from build123d import *

# Parameters (mm, degrees)
SKETCH2_R            = 39.5
BOSS_EXTRUDE1_DEPTH  = 1
SKETCH4_R            = 41.25
BOSS_EXTRUDE2_DEPTH  = 1
SKETCH5_R            = 42
BOSS_EXTRUDE3_DEPTH  = 7
SKETCH6_R            = 35
BOSS_EXTRUDE4_DEPTH  = 7
BOSS_EXTRUDE5_DEPTH  = 3
CIRPATTERN1_COUNT    = 12
SKETCH8_R            = 15
BOSS_EXTRUDE6_DEPTH  = 10
SKETCH9_W            = 24
SKETCH9_H            = 40
BOSS_EXTRUDE7_DEPTH  = 42
BOSS_EXTRUDE8_START  = -24
BOSS_EXTRUDE8_DEPTH  = 24
SKETCH11_R           = 15
BOSS_EXTRUDE9_DEPTH  = 10
BOSS_EXTRUDE10_START = 10
SKETCH12_R           = 15
BOSS_EXTRUDE10_DEPTH = 10


with BuildPart() as part:
    # Sketch1 → Revolve1 (revolve)
    with BuildSketch(Plane.XY):
        with BuildLine():
            Line((0, 0), (-35, 0))
            ThreePointArc((-35, 0), (-39.657515479, -9.46062113), (-40, -20))
            Line((-40, -20), (0, -20))
            Line((0, -20), (0, 0))
        make_face()
    revolve(axis=Axis((0, 0, 0), (0, -1, 0)))

    # Sketch2 → Boss-Extrude1 (add)
    with BuildSketch(Plane.XZ.offset(20)):
        Circle(SKETCH2_R)
    extrude(amount=BOSS_EXTRUDE1_DEPTH)

    # Sketch3 → Revolve3 (revolve)
    with BuildSketch(Plane(origin=(0, 0, 0), x_dir=(0, 0, -1), z_dir=(1, 0, 0)), mode=Mode.PRIVATE) as revolve3_sk:
        with BuildLine():
            Line((0, -21), (-40, -21))
            ThreePointArc((-40, -21), (-42.384109041, -30.861589096), (-42, -41))
            Line((-42, -41), (0, -41))
            Line((0, -41), (0, -21))
        make_face()
    revolve(revolve3_sk.sketch.rotate(Axis((0, -21, 0), (0, -1, 0)), 90), axis=Axis((0, -21, 0), (0, -1, 0)))

    # Sketch4 → Boss-Extrude2 (add)
    with BuildSketch(Plane.XZ.offset(41)):
        with Locations(Location((0, 0, 0), (0, 0, 270))):
            Circle(SKETCH4_R)
    extrude(amount=BOSS_EXTRUDE2_DEPTH)

    # Sketch5 → Boss-Extrude3 (add)
    with BuildSketch(Plane.XZ.offset(42)):
        with Locations(Location((0, 0, 0), (0, 0, 270))):
            Circle(SKETCH5_R)
    extrude(amount=BOSS_EXTRUDE3_DEPTH)

    # Sketch6 → Boss-Extrude4 (add)
    with BuildSketch(Plane.XZ.offset(49)):
        with Locations(Location((0, 0, 0), (0, 0, 270))):
            Circle(SKETCH6_R)
    extrude(amount=BOSS_EXTRUDE4_DEPTH)

    # Sketch7 → Boss-Extrude5 (add)
    with BuildSketch(Plane.XZ.offset(49)):
        Polygon((36.25, 0), (37.375, -1.948557159), (39.625, -1.948557159), (40.75, 0), (39.625, 1.948557159), (37.375, 1.948557159), align=None)
        Polygon((37.952350269, 0.948557159), (37.404700538, 0), (37.952350269, -0.948557159), (39.047649731, -0.948557159), (39.595299462, 0), (39.047649731, 0.948557159), align=None, mode=Mode.SUBTRACT)
    boss_extrude5 = extrude(amount=BOSS_EXTRUDE5_DEPTH)

    # CirPattern1: Boss-Extrude5 ×12 about axis
    cirpattern1_axis = Axis((0, 0, 0), (0, 1, 0))
    for i in range(1, CIRPATTERN1_COUNT):
        add(boss_extrude5.rotate(cirpattern1_axis, i * 360 / CIRPATTERN1_COUNT))

    # Sketch8 → Boss-Extrude6 (add)
    with BuildSketch(Plane.XZ.offset(56)):
        with Locations(Location((0, 0, 0), (0, 0, 270))):
            Circle(SKETCH8_R)
    extrude(amount=BOSS_EXTRUDE6_DEPTH)

    # Sketch9 → Boss-Extrude7 (add)
    with BuildSketch(Plane(origin=(0, 0, 0), x_dir=(1, 0, 0), z_dir=(0, 1, 0))):
        Rectangle(SKETCH9_W, SKETCH9_H)
    extrude(amount=BOSS_EXTRUDE7_DEPTH)

    # Sketch10 → Boss-Extrude8 (add)
    with BuildSketch(Plane(origin=(12, 0, 0), x_dir=(0, 0, -1), z_dir=(1, 0, 0)).offset(BOSS_EXTRUDE8_START)):
        with BuildLine():
            Line((-20, 42), (20, 42))
            ThreePointArc((20, 42), (0, 62), (-20, 42))
        make_face()
    extrude(amount=BOSS_EXTRUDE8_DEPTH)

    # Sketch11 → Boss-Extrude9 (add)
    with BuildSketch(Plane(origin=(12, 0, 0), x_dir=(0, 0, -1), z_dir=(1, 0, 0))):
        with Locations(Location((0, 42, 0), (0, 0, 180))):
            Circle(SKETCH11_R)
    extrude(amount=BOSS_EXTRUDE9_DEPTH)

    # Sketch12 → Boss-Extrude10 (add)
    with BuildSketch(Plane.ZY.offset(12).offset(BOSS_EXTRUDE10_START)):
        with Locations((0, 42)):
            Circle(SKETCH12_R)
    extrude(amount=-BOSS_EXTRUDE10_DEPTH)


solid = part.part
The model under review builds one solid part; all positions refer to its coordinate system, in mm. A direction names the side the tool comes from. Coordinates: 2 decimals unless noted, no trailing zeros. Answer as a JSON object with one key per item and string values. Group by question number.
1. To check wall thickness, follow probe 1 along Y at (x, z) = (-9, 0); probe 2 along Y at (x, z) = (32.5, -12); probe 3 along X at (y, z) = (8, -1.5). State the ranges of each line that lie inside material, in increasing order.
2. Machinability: for faces 1 (the face through (15, 0, 0)), 2 (the face through (0, 21, -20)), 3 (the face through (0.66, -60.93, 14.985)), 4 (the face through (-17.07, 56.872, -1.953)), 5 (the face through (-33.7, -52, -20.5)), which of the approach directions +Z, -Z, +X, -X, +Y, -Y give a long, thin tool a straight path to every point of the face, cutting with its end or side? Answer none if there is none.
3. Clearance check with flat-ended pins moving along their axes: pin 1 Ø1.2 at (x, y) = (-38.5, -50) entering from +Z; pin 2 Ø4 at (y, z) = (-3.5, 8.5) entering from -X; pin 3 Ø4 at (y, z) = (-45.5, 11.5) entering from +X. State where each tip first meets the part, or that it passes through.
Findings:
{
 "1": {"probe 1": "-66 to 62", "probe 2": "-56 to 0", "probe 3": "-12 to 12"},
 "2": {"face 1": "none", "face 2": "-Z, +X, -X, +Y", "face 3": "-Y", "face 4": "-X", "face 5": "-Z, -X, -Y"},
 "3": {"pin 1": "z = 1.95", "pin 2": "x = -37.45", "pin 3": "x = 40.91"}
}
